Could you check a few things on this model? Use its own coordinates, in mm. A direction names the side the tool comes from. Give positions to 0.01 mm unless a question says otherwise; leave off trailing zeros. Write each loop counter-clockwise with the first axis right and the second up, starting at its lowest first coordinate (ties: lowest second). Pieces come first, ordered by that corner, then holes. Notation, with made-up numbers: (54.5, 84.25) - (75.5, 84.25) arc R24 ccw to (75.5, 120.25) - close; hole circle Ø9 at (77.5, -5). An arc over 180 degrees is marked (long way). Answer as CSV lines item,"result". Start each with the question number.
Q1. On a 3-axis mill with a long thin cutter (end or side, diameter ignored), from which of +Z, -Z, +X, -X, +Y, -Y can I reach the whole of each face in a straight line? I mean faces 1 (the face through (4, 20, 0)), 2 (the face through (15, 0, 0)). Say none if no direction works.
Q2. If I drill on line 1 along X through (y, z) = (8.5, 11); line 2 along Y through (x, z) = (-14, 0); line 3 along Z through (x, y) = (0, 33), over which ranges is the centre line in solid material (lowest first)?
Q3. Will this pin go through, and if not, where does the flat tip stop? pin 1 Ø16 at (x, z) = (-0.5, -7) entering from -Y.
Q4. Imagine slicing it at A-A on y = 10. List the corners of the cut face in (x, z) for me.
Q5. Imagine slicing it at D-D on z = 6.5. List the corners of the cut face in (x, y) for me, and give its area (3 significant figures).
Q6. Imagine slicing it at C-C on y = 4.5. List the corners of the cut face in (x, z) for me, and give its area (3 significant figures).
Q7. We'd pull the mould along Z, two halves only. Please class faces 3 (the face through (-2.43, 30.14, -2.23)), 4 (the face through (10, 10, 5)), 5 (the face through (15.07, 14.46, 0.59)), 6 (the face through (0, 24, -20)): pulls with the +Z half, pulls with the -Z half, needs draft (parallel to the pull), parting line crosses it, or undercut.
Q8. Imagine slicing it at B-B on x = 0. List the corners of the cut face in (y, z) for me.
```python
from build123d import *

# Parameters (mm, degrees)
SKETCH1_W           = 40
SKETCH1_H           = 40
BOSS_EXTRUDE1_DEPTH = 40
SKETCH2_R           = 3.3
CUT_EXTRUDE1_DEPTH  = 40
SKETCH3_W           = 20
SKETCH3_H           = 40
CUT_EXTRUDE2_DEPTH  = 40
SKETCH4_R           = 4.5
CUT_EXTRUDE3_DEPTH  = 40


with BuildPart() as part:
    # Sketch1 → Boss-Extrude1 (new body)
    with BuildSketch(Plane(origin=(0, 0, 0), x_dir=(1, 0, 0), z_dir=(0, 1, 0))):
        Rectangle(SKETCH1_W, SKETCH1_H)
    extrude(amount=BOSS_EXTRUDE1_DEPTH)

    # Sketch2 → Cut-Extrude1 (cut)
    with BuildSketch(Plane(origin=(0, 40, 0), x_dir=(1, 0, 0), z_dir=(0, 1, 0))):
        Circle(SKETCH2_R)
    extrude(amount=-CUT_EXTRUDE1_DEPTH, mode=Mode.SUBTRACT)

    # Sketch3 → Cut-Extrude2 (cut)
    with BuildSketch(Plane.XY.offset(20)):
        Rectangle(SKETCH3_W, SKETCH3_H)
    extrude(amount=-CUT_EXTRUDE2_DEPTH, mode=Mode.SUBTRACT)

    # Sketch4 → Cut-Extrude3 (cut)
    with BuildSketch(Plane(origin=(20, 0, 0), x_dir=(0, 0, -1), z_dir=(1, 0, 0))):
        with Locations((0, 10)):
            Circle(SKETCH4_R)
    extrude(amount=-CUT_EXTRUDE3_DEPTH, mode=Mode.SUBTRACT)


solid = part.part
```
Conclusion:
1,face 1,"+Z, -Z, -Y"
1,face 2,"+Z, -Z, +X, -X, -Y"
2,line 1,"-20 to -10, 10 to 20"
2,line 2,"0 to 5.5, 14.5 to 40"
2,line 3,"-20 to -3.3, 3.3 to 20"
3,pin 1,"y = 20"
4,outline,"(-20, -20) - (-10, -20) - (-10, -4.5) - (-20, -4.5) - close; (-20, 4.5) - (-10, 4.5) - (-10, 20) - (-20, 20) - close; (10, -20) - (20, -20) - (20, -4.5) - (10, -4.5) - close; (10, 4.5) - (20, 4.5) - (20, 20) - (10, 20) - close"
5,outline,"(-20, 0) - (-10, 0) - (-10, 20) - (10, 20) - (10, 0) - (20, 0) - (20, 40) - (-20, 40) - close"
5,area,"1,200 mm^2"
6,outline,"(-20, -20) - (-10, -20) - (-10, 20) - (-20, 20) - close; (10, -20) - (20, -20) - (20, 20) - (10, 20) - close"
6,area,"800 mm^2"
7,face 3,"undercut"
7,face 4,"needs draft"
7,face 5,"undercut"
7,face 6,"pulls with the -Z half"
8,outline,"(20, -20) - (40, -20) - (40, -3.3) - (20, -3.3) - close; (20, 3.3) - (40, 3.3) - (40, 20) - (20, 20) - close"
